The model under review builds one solid part; all positions refer to its coordinate system, in mm. A direction names the side the tool comes from. Give positions to 0.01 mm unless a question says otherwise; leave off trailing zeros. Loops run counter-clockwise (first coordinate to the right, second up) from the corner with the lowest first, then second, coordinate; pieces in that order, holes last. Notation, with made-up numbers: M 81,10 L 93,10 A21 cw 93,43 Z; hole C 78,17.25 d4. An arc over 180 degrees is marked long. One line per item, written item: value. Start each with the question number.
Q1. To check wall thickness, follow line 1 along Z through (x, y) = (-2.55, 1.75); line 2 along Y through (x, z) = (1.85, -0.85); line 3 along Y through (x, z) = (-1.45, -0.25). State the ranges of each line that lie inside material, in increasing order. Write a range as from..to.
Q2. We need section A-A on y = -3.75. Write out the cut boundary in (x, z), plus the area to 3 significant figures.
Q3. For faces 5 (the face through (2, 2.5, -1)), 6 (the face through (1, 0, -1)), list the 3-axis set-ups (+Z, -Z, +X, -X, +Y, -Y) from which the entire face can be reached by the end or side of a thin tool; tool diameter is ignored.
Q4. For pin 1 (2 mm diameter, centred on x = 1.5, y = -4.5, fed in from -Z), flat-tipped, find the tip position at first contact; note if it passes through.
Q5. Mouldability with a two-part tool opening along Z and no side actions: class faces 1 (the face through (-0.225, -5.423, 0.715)), 2 (the face through (1.89, 1.76, -0.25)), 3 (the face through (0, -11, 0)), 4 (the face through (0, 1, 0)) as released by +Z, released by -Z, zero draft, split by the parting line, or undercut.
```python
from build123d import *

# Parameters (mm, degrees)
BOSS_EXTRUDE2_DEPTH = 2.5
SKETCH5_R           = 1.905
CUT_EXTRUDE1_DEPTH  = 1.5
SKETCH6_R           = 0.75
BOSS_EXTRUDE3_DEPTH = 11


# Read off the part's stored shape, not the designer's step: Boss-Extrude2
with BuildPart() as part:
    # Boss-Extrude2 outline → Boss-Extrude2 (new body)
    with BuildSketch(Plane(origin=(0, 0, 0), x_dir=(1, 0, 0), z_dir=(0, 1, 0))):
        with BuildLine():
            ThreePointArc((-0.444105945, -2.466402753), (-0.203951755, -2.501641146), (0.038487797, -2.513424302))
            Line((0.038487797, -2.513424302), (0.038487797, -3.013424302))
            Line((0.038487797, -3.013424302), (0.337525902, -2.495475109))
            ThreePointArc((0.337525902, -2.495475109), (0.429573959, -2.482645153), (0.521081538, -2.466402753))
            Line((0.521081538, -2.466402753), (0.96553878, -2.866593851))
            Line((0.96553878, -2.866593851), (1.089885816, -2.28158704))
            ThreePointArc((1.089885816, -2.28158704), (1.173464046, -2.240940612), (1.255473747, -2.197215774))
            Line((1.255473747, -2.197215774), (1.801843553, -2.440475285))
            Line((1.801843553, -2.440475285), (1.739327566, -1.845675398))
            ThreePointArc((1.739327566, -1.845675398), (1.80625475, -1.781191255), (1.870738892, -1.714264071))
            Line((1.870738892, -1.714264071), (2.46553878, -1.776780059))
            Line((2.46553878, -1.776780059), (2.222279269, -1.230410253))
            ThreePointArc((2.222279269, -1.230410253), (2.266004107, -1.148400551), (2.306650534, -1.064822321))
            Line((2.306650534, -1.064822321), (2.891657345, -0.940475285))
            Line((2.891657345, -0.940475285), (2.491466248, -0.496018043))
            ThreePointArc((2.491466248, -0.496018043), (2.507708648, -0.404510464), (2.520538604, -0.312462408))
            Line((2.520538604, -0.312462408), (3.038487797, -0.013424302))
            Line((3.038487797, -0.013424302), (2.520538604, 0.285613804))
            ThreePointArc((2.520538604, 0.285613804), (2.507708648, 0.377661861), (2.491466248, 0.46916944))
            Line((2.491466248, 0.46916944), (2.891657345, 0.913626681))
            Line((2.891657345, 0.913626681), (2.306650534, 1.037973718))
            ThreePointArc((2.306650534, 1.037973718), (2.266004107, 1.121551948), (2.222279269, 1.203561649))
            Line((2.222279269, 1.203561649), (2.46553878, 1.749931455))
            Line((2.46553878, 1.749931455), (1.870738892, 1.687415468))
            ThreePointArc((1.870738892, 1.687415468), (1.80625475, 1.754342652), (1.739327566, 1.818826794))
            Line((1.739327566, 1.818826794), (1.801843553, 2.413626681))
            Line((1.801843553, 2.413626681), (1.255473747, 2.170367171))
            ThreePointArc((1.255473747, 2.170367171), (1.173464046, 2.214092009), (1.089885816, 2.254738436))
            Line((1.089885816, 2.254738436), (0.96553878, 2.839745247))
            Line((0.96553878, 2.839745247), (0.521081538, 2.439554149))
            ThreePointArc((0.521081538, 2.439554149), (0.429573959, 2.45579655), (0.337525902, 2.468626506))
            Line((0.337525902, 2.468626506), (0.038487797, 2.986575698))
            Line((0.038487797, 2.986575698), (-0.260550309, 2.468626506))
            ThreePointArc((-0.260550309, 2.468626506), (-0.352598366, 2.45579655), (-0.444105945, 2.439554149))
            Line((-0.444105945, 2.439554149), (-0.888563187, 2.839745247))
            Line((-0.888563187, 2.839745247), (-1.012910223, 2.254738436))
            ThreePointArc((-1.012910223, 2.254738436), (-1.096488453, 2.214092009), (-1.178498154, 2.170367171))
            Line((-1.178498154, 2.170367171), (-1.72486796, 2.413626681))
            Line((-1.72486796, 2.413626681), (-1.662351973, 1.818826794))
            ThreePointArc((-1.662351973, 1.818826794), (-1.729279156, 1.754342651), (-1.793763299, 1.687415468))
            Line((-1.793763299, 1.687415468), (-2.388563187, 1.749931455))
            Line((-2.388563187, 1.749931455), (-2.145303676, 1.203561649))
            ThreePointArc((-2.145303676, 1.203561649), (-2.189028514, 1.121551948), (-2.229674941, 1.037973718))
            Line((-2.229674941, 1.037973718), (-2.814681752, 0.913626681))
            Line((-2.814681752, 0.913626681), (-2.414490654, 0.46916944))
            ThreePointArc((-2.414490654, 0.46916944), (-2.430733055, 0.377661861), (-2.443563011, 0.285613804))
            Line((-2.443563011, 0.285613804), (-2.961512203, -0.013424302))
            Line((-2.961512203, -0.013424302), (-2.443563011, -0.312462408))
            ThreePointArc((-2.443563011, -0.312462408), (-2.430733055, -0.404510465), (-2.414490654, -0.496018043))
            Line((-2.414490654, -0.496018043), (-2.814681752, -0.940475285))
            Line((-2.814681752, -0.940475285), (-2.229674941, -1.064822321))
            ThreePointArc((-2.229674941, -1.064822321), (-2.189028514, -1.148400551), (-2.145303676, -1.230410253))
            Line((-2.145303676, -1.230410253), (-2.388563187, -1.776780059))
            Line((-2.388563187, -1.776780059), (-1.793763299, -1.714264071))
            ThreePointArc((-1.793763299, -1.714264071), (-1.729279156, -1.781191255), (-1.662351973, -1.845675398))
            Line((-1.662351973, -1.845675398), (-1.72486796, -2.440475285))
            Line((-1.72486796, -2.440475285), (-1.178498154, -2.197215774))
            ThreePointArc((-1.178498154, -2.197215774), (-1.096488453, -2.240940612), (-1.012910223, -2.28158704))
            Line((-1.012910223, -2.28158704), (-0.888563187, -2.866593851))
            Line((-0.888563187, -2.866593851), (-0.444105945, -2.466402753))
        make_face()
    extrude(amount=BOSS_EXTRUDE2_DEPTH)

    # Sketch5 → Cut-Extrude1 (cut)
    with BuildSketch(Plane(origin=(0, 2.5, 0), x_dir=(1, 0, 0), z_dir=(0, 1, 0))):
        with Locations(Location((0, 0, 0), (0, 0, 270))):
            Circle(SKETCH5_R)
    extrude(amount=-CUT_EXTRUDE1_DEPTH, mode=Mode.SUBTRACT)

    # Sketch6 → Boss-Extrude3 (add)
    with BuildSketch(Plane.XZ):
        with Locations(Location((0, 0, 0), (0, 0, 90))):
            Circle(SKETCH6_R)
    extrude(amount=BOSS_EXTRUDE3_DEPTH)


solid = part.part
```
Solved:
1. line 1: -0.97..-0.62, -0.22..0.25, 0.65..1
1. line 2: 0..2.5
1. line 3: 0..1
2. outline: C 0,0 d1.5
2. area: 1.77 mm2
3. face 5: +Z, -Z, +X, -X, +Y
3. face 6: -Y
4. pin 1: z = -0.56
5. face 1: split by the parting line
5. face 2: undercut
5. face 3: zero draft
5. face 4: undercut
